Part model, mm, in its own coordinate system. A direction names the side the tool comes from. Give positions to 0.01 mm unless a question says otherwise; leave off trailing zeros. Loops run counter-clockwise (first coordinate to the right, second up) from the corner with the lowest first, then second, coordinate; pieces in that order, holes last. Notation, with made-up numbers: M 71.25,73.5 L 117.25,73.5 A20 cw 117.25,103.5 Z; hole C 7.25,87 d3. An arc over 180 degrees is marked long. Put each result on its own line as item: value. Start each with the question number.
```python
from build123d import *

# Parameters (mm, degrees)
SKETCH1_R           = 7.5
BOSS_EXTRUDE1_DEPTH = 45
SKETCH2_R           = 1.5
BOSS_EXTRUDE2_DEPTH = 15
SKETCH3_R           = 3.389534101
CUT_EXTRUDE1_DEPTH  = 7.5
SKETCH4_R           = 13.089152616
CUT_EXTRUDE2_DEPTH  = 5


with BuildPart() as part:
    # Sketch1 → Boss-Extrude1 (new body)
    with BuildSketch(Plane(origin=(0, 0, 0), x_dir=(0, 0, -1), z_dir=(1, 0, 0))):
        with Locations((-35.817726835, 20.099436521)):
            Circle(SKETCH1_R)
    extrude(amount=BOSS_EXTRUDE1_DEPTH)

    # Sketch2 → Boss-Extrude2 (add)
    with BuildSketch(Plane(origin=(45, 0, 0), x_dir=(0, 0, -1), z_dir=(1, 0, 0))):
        with Locations((-35.817726835, 20.099436521)):
            Circle(SKETCH2_R)
    extrude(amount=BOSS_EXTRUDE2_DEPTH)

    # Sketch3 → Cut-Extrude1 (cut)
    with BuildSketch(Plane(origin=(60, 0, 0), x_dir=(0, 0, -1), z_dir=(1, 0, 0))):
        with Locations((-35.761209842, 20.149750274)):
            Circle(SKETCH3_R)
    extrude(amount=-CUT_EXTRUDE1_DEPTH, mode=Mode.SUBTRACT)

    # Sketch4 → Cut-Extrude2 (cut)
    with BuildSketch(Plane.ZY):
        with Locations((34.849696462, 19.463840008)):
            Circle(SKETCH4_R)
    extrude(amount=-CUT_EXTRUDE2_DEPTH, mode=Mode.SUBTRACT)


solid = part.part
```
1) Which spindle directions (+Z, -Z, +X, -X, +Y, -Y) get a long thin tool onto all of the face, cutting with end or side? Do faces 1 (the cylindrical face through (48.698, 21.113, 36.923)), 2 (the flat face through (5, 20, 36)). Say none if no direction does.
2) Pin check, flat tips, straight feed: pin 1 Ø4 at (y, z) = (16, 32.5) entering from +X; pin 2 Ø5 at (x, y) = (15.5, 25) entering from +Z; pin 3 Ø8 at (x, z) = (44.5, 40) entering from -Y. Stop position of each tip, or through.
3) Wall check: L1, parallel to X at y = 23.25, z = 32.5; L2, parallel to Z at x = 43, y = 20; L3, parallel to Z at x = 44, y = 23.75. Give the ranges that are in metal, low to high.
4) Band-saw the part on A-A on z = 30.5. Give the cut face in (x, y).
5) Band-saw the part on B-B on y = 15.25. Give the cut face in (x, z), then the cut area to 3 significant figures.
6) Band-saw the part on C-C on x = 29. Give the cut face in (y, z), then the cut area to 3 significant figures.
Evaluation:
1. face 1: +X
1. face 2: +Z, -Z, -X, +Y, -Y
2. pin 1: x = 45
2. pin 2: z = 42.92
2. pin 3: y = 12.6
3. L1: 5 to 45
3. L2: 28.32 to 43.32
3. L3: 29.27 to 42.37
4. outline: M 5,14.81 L 45,14.81 L 45,25.39 L 5,25.39 Z
5. outline: M 5,30.1 L 45,30.1 L 45,41.54 L 5,41.54 Z
5. area: 458 mm2
6. outline: C 20.1,35.82 d15
6. area: 177 mm2
